```python
from build123d import *

# Parameters (mm, degrees)
SKETCH4_OUTSIDE_W = 13.574
SKETCH4_OUTSIDE_H = 13.574
CUT_KEY_DEPTH     = 14.2


with BuildPart() as part:
    # Sketch6 → body (revolve)
    with BuildSketch(Plane.XY):
        with BuildLine():
            Line((0.992845254, 13.2), (2.25, 13.2))
            Line((2.25, 13.2), (3.25, 11.45255235))
            ThreePointArc((3.25, 11.45255235), (3.263671492, 10.119347494), (2.752432371, 8.887983756))
            ThreePointArc((2.752432371, 8.887983756), (2.616668661, 8.494453666), (2.697011723, 8.085989826))
            ThreePointArc((2.697011723, 8.085989826), (3.268727336, 7.226263337), (4.041451884, 6.541511445))
            Line((4.041451884, 6.541511445), (4.041451884, 5.479056191))
            Line((4.041451884, 5.479056191), (3, 5.2))
            Line((3, 5.2), (3, 2.4))
            Line((3, 2.4), (2.746726841, 0.337255649))
            Line((2.746726841, 0.337255649), (2.409471192, 0))
            Line((2.409471192, 0), (0, 0))
            Line((0, 0), (0, 13.2))
            ThreePointArc((0, 13.2), (0.351023806, 13.054601179), (0.496422627, 12.703577373))
            ThreePointArc((0.496422627, 12.703577373), (0.641821448, 13.054601179), (0.992845254, 13.2))
        make_face()
    revolve(axis=Axis((0, 0, 0), (0, 1, 0)))

    # Sketch4 outside → cut-key (cut, through all)
    with BuildSketch(Plane(origin=(0, 0, 0), x_dir=(1, 0, 0), z_dir=(0, 1, 0))):
        Rectangle(SKETCH4_OUTSIDE_W, SKETCH4_OUTSIDE_H)
        Polygon((3.5, -2.020725942), (3.5, 2.020725942), (0, 4.041451884), (-3.5, 2.020725942), (-3.5, -2.020725942), (0, -4.041451884), align=None, mode=Mode.SUBTRACT)
    extrude(amount=CUT_KEY_DEPTH, mode=Mode.SUBTRACT)


solid = part.part
```
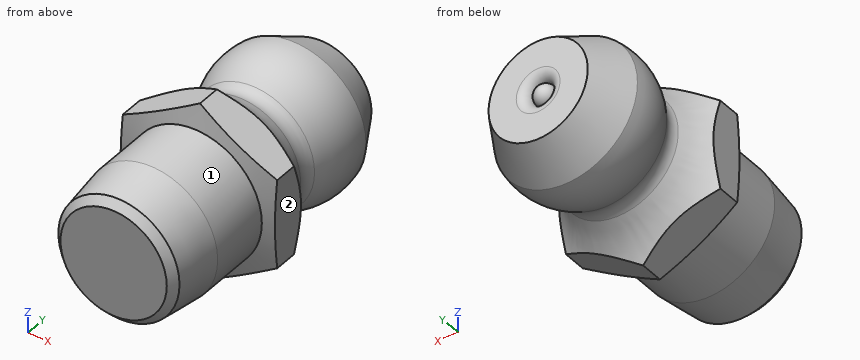
For this review, take the finished solid that the model builds, in its own axes (mm). Face numbers are marked on the shaded views. A direction names the side the tool comes from. Give positions to 0.01 mm unless a question says otherwise; leave off trailing zeros. Write each loop counter-clockwise with the first axis right and the second up, starting at its lowest first coordinate (ties: lowest second). Pieces come first, ordered by that corner, then holes.
Item 1: Machinability: for the marked faces 1 and 2, which of the approach directions +Z, -Z, +X, -X, +Y, -Y give a long, thin tool a straight path to every point of the face, cutting with its end or side? Answer none if there is none.
Item 2: Take a section at B-B (y = 3.75). Give the boundary of the cut face in (x, z).
Item 3: Insertion check: P1, Ø4, axis at x = 2.5, z = -1.5, coming from the -Y side. The pin has a flat end and moves straight along its axis. Give the tip position at first contact, or say it passes through.
Item 4: Take a section at C-C (y = 8.75). Give the boundary of the cut face in (x, z), and give its area (3 significant figures).
Item 5: Wall thickness on probe 1 along X at (y, z) = (11.25, -0.5); probe 2 along Z at (x, y) = (-0.5, 6.5); probe 3 along Z at (x, y) = (-2.25, 8.5): over which ranges is each line inside the solid? List them lowest first.
Item 6: Take a section at A-A (z = 0). Give the boundary of the cut face in (x, y).
Established:
1. face 1: -Y
1. face 2: +Z, -Z, +X, +Y, -Y
2. outline: circle Ø6 at (0, 0)
3. P1: stops at y = 0
4. outline: circle Ø5.36 at (0, 0)
4. area: 22.5 mm2
5. probe 1: x = -3.25 to 3.25
5. probe 2: z = -3.75 to 3.75
5. probe 3: z = -1.34 to 1.34
6. outline: (-3.5, 5.33) - (-3, 5.2) - (-3, 2.4) - (-2.75, 0.34) - (-2.41, 0) - (2.41, 0) - (2.75, 0.34) - (3, 2.4) - (3, 5.2) - (3.5, 5.33) - (3.5, 6.98) arc R4 cw to (2.7, 8.09) arc R0.8 cw to (2.75, 8.89) arc R3.32 ccw to (3.25, 11.45) - (2.25, 13.2) - (0.99, 13.2) arc R0.5 ccw to (0.5, 12.7) arc R0.5 ccw to (-0.5, 12.7) arc R0.5 ccw to (-0.99, 13.2) - (-2.25, 13.2) - (-3.25, 11.45) arc R3.32 ccw to (-2.75, 8.89) arc R0.8 cw to (-2.7, 8.09) arc R4 cw to (-3.5, 6.98) - close
